Verification items for the finished model (mm, model axes). A direction names the side the tool comes from. Coordinates: 2 decimals unless noted, no trailing zeros. Loops run counter-clockwise (first coordinate to the right, second up) from the corner with the lowest first, then second, coordinate; pieces in that order, holes last. Notation, with made-up numbers: M -11,47.5 L 40,47.5 A20 ccw 40,60.5 Z; hole C 65,-0.5 d4. An arc over 180 degrees is marked long. Write item = value, one per line. Start each with the question number.
```python
from build123d import *

# Parameters (mm, degrees)
BOSS_EXTRUDE1_START = 10
BOSS_EXTRUDE1_DEPTH = 150
CUT_EXTRUDE1_START  = -38
SKETCH3_R           = 23
CUT_EXTRUDE1_DEPTH  = 81.301270189
CUT_EXTRUDE2_START  = -33.3
SKETCH4_R           = 5
CUT_EXTRUDE2_DEPTH  = 4.7


with BuildPart() as part:
    # Sketch1 → Boss-Extrude1 (new body)
    with BuildSketch(Plane(origin=(0, 0, 0), x_dir=(1, 0, 0), z_dir=(0, 1, 0)).offset(BOSS_EXTRUDE1_START)):
        Polygon((0, 50), (-43.301270189, 25), (-43.301270189, -25), (0, -50), (43.301270189, -25), (43.301270189, 25), align=None)
    extrude(amount=BOSS_EXTRUDE1_DEPTH)

    # Sketch3 → Cut-Extrude1 (cut)
    with BuildSketch(Plane(origin=(0, 0, 0), x_dir=(0, 0, -1), z_dir=(1, 0, 0)).offset(CUT_EXTRUDE1_START)):
        with Locations((0, 23)):
            Circle(SKETCH3_R)
    cut_extrude1 = extrude(amount=-CUT_EXTRUDE1_DEPTH, mode=Mode.SUBTRACT)

    # Sketch4 → Cut-Extrude2 (cut)
    with BuildSketch(Plane(origin=(0, 0, 0), x_dir=(0, 0, -1), z_dir=(1, 0, 0)).offset(CUT_EXTRUDE2_START)):
        with Locations((0, 23)):
            Circle(SKETCH4_R)
    cut_extrude2 = extrude(amount=-CUT_EXTRUDE2_DEPTH, mode=Mode.SUBTRACT)

    # Mirror4: Cut-Extrude1, Cut-Extrude2 across plane
    add(cut_extrude1.mirror(Plane(origin=(0, 0, 0), x_dir=(0, 0, 1), z_dir=(1, 0, 0))), mode=Mode.SUBTRACT)
    add(cut_extrude2.mirror(Plane(origin=(0, 0, 0), x_dir=(0, 0, 1), z_dir=(1, 0, 0))), mode=Mode.SUBTRACT)


solid = part.part
```
Q1. Sectioned sample at B-B on y = 23. Record the cut outline in (x, z).
Q2. Sectioned sample at A-A on z = 0. Record the cut outline in (x, y), plus the area to 3 significant figures.
Q3. Sectioned sample at C-C on x = 7.5. Record the cut outline in (y, z).
Q4. Sectioned sample at D-D on y = 67.5. Record the cut outline in (x, z).
Q5. Gauge pin test, flat ends, axial feed: pin 1 (5 mm diameter, centred on y = 23.5, z = -1.5, fed in from -X); pin 2 (1.5 mm diameter, centred on x = 14, y = 117, fed in from +Z); pin 3 (2 mm diameter, centred on x = 25, y = 57.5, fed in from -Z). Record the tip position at first contact, or that the pin passes through.
Q6. Scan lines: L1, parallel to Y at x = 34.3, z = 0; L2, parallel to Y at x = 39, z = 0; L3, parallel to Z at x = -39.4, y = 23. Record each from-to range of solid material in increasing order. Write a range as [from, to].
Q7. Mould release check, pull along Z, two halves, no side actions. Record for faces 1 (the face through (22, 84, -37.3)), 2 (the face through (35.62, 18.12, 1.08)), 3 (the face through (21.348, 83.95, 37.675)): +Z half, -Z half, draft (parallel to the pull), parting line (faces both ways), or undercut.
Q8. Set-up check for faces 4 (the face through (40.61, 45.99, -0.7)), 5 (the face through (-1, 160, -1)), 6 (the face through (-40.61, 45.99, -0.7)): record each of +Z, -Z, +X, -X, +Y, -Y from which the full face is reachable in a straight line by a thin tool's end or side.
Solutions:
q1.outline = M -43.3,-25 L 0,-50 L 43.3,-25 L 43.3,-23 L 38,-23 L 38,-5 L 33.3,-5 L 33.3,5 L 38,5 L 38,23 L 43.3,23 L 43.3,25 L 0,50 L -43.3,25 L -43.3,23 L -38,23 L -38,5 L -33.3,5 L -33.3,-5 L -38,-5 L -38,-23 L -43.3,-23 Z
q2.outline = M -43.3,46 L -38,46 L -38,28 L -33.3,28 L -33.3,18 L -38,18 L -38,10 L 38,10 L 38,18 L 33.3,18 L 33.3,28 L 38,28 L 38,46 L 43.3,46 L 43.3,160 L -43.3,160 Z
q2.area = 12,500 mm²
q3.outline = M 10,-45.67 L 160,-45.67 L 160,45.67 L 10,45.67 Z
q4.outline = M -43.3,-25 L 0,-50 L 43.3,-25 L 43.3,25 L 0,50 L -43.3,25 Z
q5.pin_1 = -33.3
q5.pin_2 = 42.35
q5.pin_3 = -36.14
q6.L1 = [10, 18], [28, 160]
q6.L2 = [46, 160]
q6.L3 = [-27.25, -23], [23, 27.25]
q7.face_1 = -Z half
q7.face_2 = undercut
q7.face_3 = +Z half
q8.face_4 = +X
q8.face_5 = +Z, -Z, +X, -X, +Y
q8.face_6 = -X
